Part print with two shaded views. Sizes in mm from the minimum x, y, z corner. A direction names the side the tool comes from. Round coordinates to 2 decimals unless told otherwise and drop trailing zeros. Write each loop counter-clockwise with the first axis right and the second up, starting at its lowest first coordinate (ties: lowest second). Pieces come first, ordered by that corner, then holes. Notation, with made-up numbers: (-3, 85) - (22, 85) arc R16 ccw to (22, 95) - close; hole circle Ø7 at (51, -31.75). An arc over 180 degrees is marked (long way). Use one line per item in the form item = value. Start each with the question number.
Item 1: Band-saw the part on A-A, the plane y = 12.7. List the corners of the cut face in (x, z) (3 decimals), and give its area (3 significant figures).
Item 2: Pull direction Y, two halves, no side cores. Call the marked faces 6, 7 and 8: +Y half, -Y half, draft (parallel to the pull), parting line (faces both ways), or undercut.
Item 3: Drill centre lines: L1, parallel to Y at x = 3, z = 2.1 (3 decimals); L2, parallel to X at y = 6.25, z = 2.15 (3 decimals); L3, parallel to X at y = 11.5, z = 2.1. Where is each one in solid material? Low to high.
Item 4: Band-saw the part on C-C, the plane x = 12. List the corners of the cut face in (y, z) (3 decimals), and give its area (3 significant figures).
Item 5: Tool access for the marked faces 1, 2, 3, 4 and 5: list every direction of +Z, -Z, +X, -X, +Y, -Y with a clear straight run to the whole face (end or side of a thin tool).
Item 6: Band-saw the part on D-D, the plane x = 5.75. List the corners of the cut face in (y, z) (3 decimals).
Item 7: Band-saw the part on B-B, the plane z = 2.15. List the corners of the cut face in (x, y) (3 decimals).
Item 8: Pin check, flat tips, straight feed: pin 1 (1.6 mm diameter, centred on x = 2, z = 1.5, fed in from +Y) (3 decimals); pin 2 (1 mm diameter, centred on x = 5, z = 1.5, fed in from -Y) (3 decimals); pin 3 (1.5 mm diameter, centred on x = 2.5, z = 2.5, fed in from +Y) (3 decimals); pin 4 (5 mm diameter, centred on x = 16.5, y = 11, fed in from -Z). Stop position of each tip, or through.
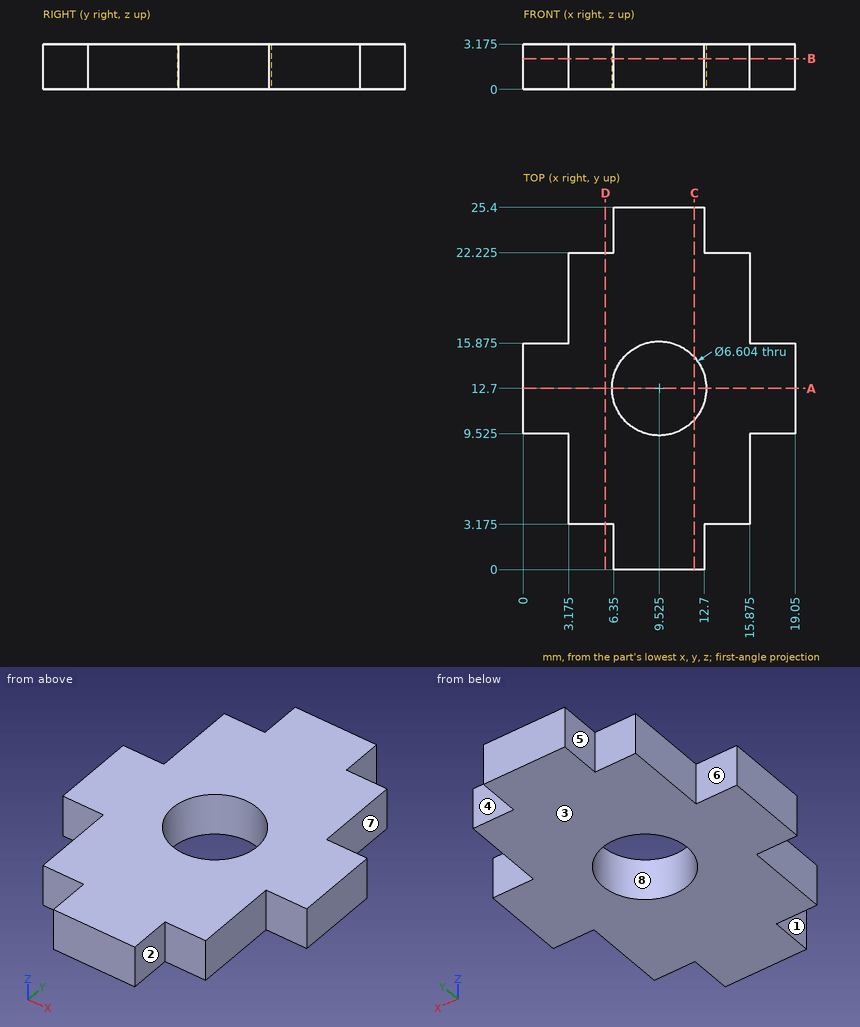
Determined:
q1.outline = (0, 0) - (6.223, 0) - (6.223, 3.175) - (0, 3.175) - close; (12.827, 0) - (19.05, 0) - (19.05, 3.175) - (12.827, 3.175) - close
q1.area = 39.5 mm²
q2.face_6 = +Y half
q2.face_7 = draft
q2.face_8 = undercut
q3.L1 = 9.525 to 15.875
q3.L2 = 3.175 to 15.875
q3.L3 = 0 to 6.45, 12.6 to 19.05
q4.outline = (0, 0) - (10.514, 0) - (10.514, 3.175) - (0, 3.175) - close; (14.886, 0) - (25.4, 0) - (25.4, 3.175) - (14.886, 3.175) - close
q4.area = 66.8 mm²
q5.face_1 = +Z, -Z, -X, -Y
q5.face_2 = +Z, -Z, +X, -Y
q5.face_3 = -Z, +X, -X, +Y, -Y
q5.face_4 = +Z, -Z, +X, +Y
q5.face_5 = +Z, -Z, -X, +Y
q6.outline = (3.175, 0) - (22.225, 0) - (22.225, 3.175) - (3.175, 3.175) - close
q7.outline = (0, 9.525) - (3.175, 9.525) - (3.175, 3.175) - (6.35, 3.175) - (6.35, 0) - (12.7, 0) - (12.7, 3.175) - (15.875, 3.175) - (15.875, 9.525) - (19.05, 9.525) - (19.05, 15.875) - (15.875, 15.875) - (15.875, 22.225) - (12.7, 22.225) - (12.7, 25.4) - (6.35, 25.4) - (6.35, 22.225) - (3.175, 22.225) - (3.175, 15.875) - (0, 15.875) - close; hole circle Ø6.604 at (9.525, 12.7)
q8.pin_1 = 15.875
q8.pin_2 = 3.175
q8.pin_3 = 22.225
q8.pin_4 = 0
